```python
from build123d import *

# Parameters (mm, degrees)
F0_W     = 914.4
F0_H     = 558.8
F1_DEPTH = 285.75
F2_W     = 876.3
F2_H     = 260.35
F3_DEPTH = 285.751
F4_W     = 158.75
F4_H     = 558.8
F5_DEPTH = 19.05
F6_W     = 158.75
F6_H     = 558.8
F7_DEPTH = 19.05


with BuildPart() as f1:
    # F0 (on Front) → F1 (new body)
    with BuildSketch(Plane.XZ):
        with Locations((-544.727786, 279.4)):
            Rectangle(F0_W, F0_H)
    extrude(amount=F1_DEPTH)

    # F2 (on face) → F3 (cut, through all)
    with BuildSketch(Plane.XZ.offset(285.75)):
        with Locations((-544.727786, 130.175)):
            Rectangle(F2_W, F2_H)
        with Locations((-544.727786, 409.575)):
            Rectangle(F2_W, F2_H)
    extrude(amount=-F3_DEPTH, mode=Mode.SUBTRACT)

    # F4 (on face) → F5 (cut, through all)
    with BuildSketch(Plane.YZ.offset(-87.527786)):
        with Locations((-142.875, 279.4)):
            Rectangle(F4_W, F4_H)
    extrude(amount=-F5_DEPTH, mode=Mode.SUBTRACT)

    # F6 (on face) → F7 (cut, through all)
    with BuildSketch(Plane(origin=(-1001.927786, 0, 0), x_dir=(0, -1, 0), z_dir=(-1, 0, 0))):
        with Locations((142.875, 279.4)):
            Rectangle(F6_W, F6_H)
    extrude(amount=-F7_DEPTH, mode=Mode.SUBTRACT)


solid = f1.part
```
Can you work these out from the model? Positions are in its coordinate system, mm. A direction names the side the tool comes from. Give positions to 0.01 mm unless a question says otherwise; leave off trailing zeros. Loops run counter-clockwise (first coordinate to the right, second up) from the corner with the lowest first, then second, coordinate; pieces in that order, holes last. Notation, with made-up numbers: M 11,-3 L 30,-3 A13 ccw 30,18 Z; hole C 8,5 d4. An arc over 180 degrees is marked long. Answer in a Markdown table with one row per item.
1. Which directions (+Z, -Z, +X, -X, +Y, -Y) give clear straight access to the entire face, cutting with the end or side of a thin tool? Please do faces 1 (the flat face through (-982.878, -142, 270)), 2 (the flat face through (-106.578, -144, 549)), 3 (the flat face through (-551, -145, 260.35)).
Taken from the geometry:
| item | result |
|---|---|
| face 1 | +Z, -Z, -X |
| face 2 | +Z, -Z, +X |
| face 3 | -Z, +Y, -Y |
2. Suppose I cut it at A-A on y = -108. Write out the boundary of the cut face in (x, z).
Taken from the geometry:
| item | result |
|---|---|
| outline | M -982.88,260.35 L -106.58,260.35 L -106.58,279.4 L -982.88,279.4 Z; M -982.88,539.75 L -106.58,539.75 L -106.58,558.8 L -982.88,558.8 Z |
3. Suppose I cut it at C-C on x = -614.5. Write out the boundary of the cut face in (y, z), plus the area to 3 significant figures.
Taken from the geometry:
| item | result |
|---|---|
| outline | M -285.75,260.35 L 0,260.35 L 0,279.4 L -285.75,279.4 Z; M -285.75,539.75 L 0,539.75 L 0,558.8 L -285.75,558.8 Z |
| area | 10,900 mm² |
4. If I drill on line 1 along Z through (x, y) = (-670, -193); line 2 along X through (y, z) = (-227, 345), over which ranges is the centre line in solid material (lowest first)?
Taken from the geometry:
| item | result |
|---|---|
| line 1 | z = 260.35 to 279.4, 539.75 to 558.8 |
| line 2 | x = -1001.93 to -982.88, -106.58 to -87.53 |
5. For pin 1 Ø9.5 at (y, z) = (-161.5, 550.5) entering from -X; pin 2 Ø9.5 at (y, z) = (-162.5, 267) entering from +X; pin 3 Ø10 at (x, y) = (-835.5, -171.5) entering from -Z, each with a flat end and sliding along its axis, tell me the tip position at first contact or that it passes through.
Taken from the geometry:
| item | result |
|---|---|
| pin 1 | stops at x = -982.88 |
| pin 2 | stops at x = -106.58 |
| pin 3 | stops at z = 260.35 |
6. Suppose I cut it at B-B on z = 165. Write out the boundary of the cut face in (x, y), plus the area to 3 significant figures.
Taken from the geometry:
| item | result |
|---|---|
| outline | M -1001.93,-285.75 L -982.88,-285.75 L -982.88,-222.25 L -1001.93,-222.25 Z; M -1001.93,-63.5 L -982.88,-63.5 L -982.88,0 L -1001.93,0 Z; M -106.58,-285.75 L -87.53,-285.75 L -87.53,-222.25 L -106.58,-222.25 Z; M -106.58,-63.5 L -87.53,-63.5 L -87.53,0 L -106.58,0 Z |
| area | 4,840 mm² |
7. Thinking about a two-plate mould opening in Y: for faces 4 (the flat face through (-750, 0, 550)), 5 (the flat face through (-551, -145, 539.75)), 6 (the flat face through (-97, -222.25, 275)), which applies, released by +Y, released by -Y, zero draft, split by the parting line, or undercut?
Taken from the geometry:
| item | result |
|---|---|
| face 4 | released by +Y |
| face 5 | zero draft |
| face 6 | undercut |
8. Suppose I cut it at D-D on z = 270. Write out the boundary of the cut face in (x, y), plus the area to 3 significant figures.
Taken from the geometry:
| item | result |
|---|---|
| outline | M -1001.93,-285.75 L -87.53,-285.75 L -87.53,-222.25 L -106.58,-222.25 L -106.58,-63.5 L -87.53,-63.5 L -87.53,0 L -1001.93,0 L -1001.93,-63.5 L -982.88,-63.5 L -982.88,-222.25 L -1001.93,-222.25 Z |
| area | 255,000 mm² |
